Here's how the part is built. I have some questions about the finished solid (model axes, mm). Round coordinates to 2 decimals unless told otherwise and drop trailing zeros. Order: outer loops, then holes, each group sorted by start corner. A loop starts at its lowest first (then second) coordinate and runs counter-clockwise, first axis right, second up. Notation, with made-up numbers: (7, 67) -> (13, 67) arc R27 ccw to (13, 104) -> close; hole circle Ø10 at (37, 57). An arc over 180 degrees is marked (long way). Use a Markdown table: item, result. Add a question column.
(1) I want a section at B-B, the plane x = -173. Please give me the cut outline in (y, z).
(2) I want a section at A-A, the plane y = 2.75. Give the number of separate pieces and of enclosed holes in the cut face, then the cut area to 3 significant figures.
(3) If I drill on probe 1 along Y at (x, z) = (-139, 6.25); probe 2 along Z at (x, y) = (-180, 3.65); probe 3 along Z at (x, y) = (152, 6.25), over which ranges is the centre line in solid material (lowest first)?
(4) I'm going to push flat-ended pins straight in: P1, Ø5.5, axis at x = -220, z = 0, coming from the +Y side; P2, Ø2, axis at x = 20, z = 0, coming from the -Y side. Where does each tip first touch, or does it pass through?
Autodesk Inventor part; units mm, degrees
ref_plane "YZ Plane" through (0, 0, 0) normal (1, 0, 0) x (0, 1, 0)
ref_plane "XZ Plane" through (0, 0, 0) normal (0, 1, 0) x (-1, 0, 0)
ref_plane "XY Plane" through (0, 0, 0) normal (0, 0, 1) x (1, 0, 0)
sketch "Skizze1" plane through (0, 0, 0) normal (1, 0, 0) x (0, 1, 0)
  line L0 (0, 0) -> (0, -7.5)
  line L1 (0, -7.5) -> (5, -7.5)
  line L2 (0, -10.5) -> (0, 10.5)
  line L3 (-2, 0) -> (12, 0)
  arc A0 (8, -7.5) -> (5, -7.5) centre (6.5, -7.5) ccw
  line L4 (8, -7.5) -> (10, -7.5)
  line L5 (10, -7.5) -> (10, 0)
  line L6 (0, 0) -> (0, 7.5)
  line L7 (0, 7.5) -> (5, 7.5)
  arc A1 (5, 7.5) -> (8, 7.5) centre (6.5, 7.5) ccw
  line L8 (8, 7.5) -> (10, 7.5)
  line L9 (10, 7.5) -> (10, 0)
  dimension "d1" = 1.5
  dimension "d2" = 15
  dimension "d3" = 10
  dimension "d4" = 3.5
extrude "Extrusion1" add sketch "Skizze1" along normal mid plane 450
chamfer "Fase1" distance 0.4 distance2 0.4 2 edges at (0, 10, 7.5) (0, 10, -7.5) measured on face at (75, 8.6667, -7.5) measured on face at (75, 10, 2.5)
chamfer "Fase2" distance 0.4 distance2 0.4 1 edges at (0, 0, 7.5) measured on face at (-75, 3.3333, 7.5)
chamfer "Fase3" distance 0.4 distance2 0.4 1 edges at (0, 0, -7.5) measured on face at (-75, 1.6667, -7.5)
sketch "Skizze2" plane through (-225, 10, -7.1) normal (0, 1, 0) x (1, 0, 0)
  line L0 (-90, -7.1) -> (540, -7.1)
  line L1 (450, 0) -> (450, -14.2)
  point P0 (225, -7.1)
  point P1 (445, -7.1)
  dimension "d16" = 5
hole "Bohrung1" at (220, 10, 0) direction (0, -1, 0) diameter 3.4 end through all counterbore diameter 6 counterbore depth 4.9
pattern_linear "Rechteckige Anordnung1" count 12 spacing 40 along (-1, 0, 0) of "Bohrung1"
properties part number "02_mgn15h_Rail_450mm" material "Edelstahl"
Taken from the geometry:
| question | item | result |
|---|---|---|
| 1 | outline | (0, -7.1) -> (0.4, -7.5) -> (5, -7.5) arc R1.5 cw to (8, -7.5) -> (9.6, -7.5) -> (10, -7.1) -> (10, 7.1) -> (9.6, 7.5) -> (8, 7.5) arc R1.5 cw to (5, 7.5) -> (0.4, 7.5) -> (0, 7.1) -> close |
| 2 | separate pieces | 1 |
| 2 | enclosed holes | 12 |
| 2 | area | 6,640 mm2 |
| 3 | probe 1 | y = 0 to 5.67, 7.33 to 10 |
| 3 | probe 2 | z = -7.5 to -1.7, 1.7 to 7.5 |
| 3 | probe 3 | z = -6.02 to 6.02 |
| 4 | P1 | stops at y = 5.1 |
| 4 | P2 | passes through |
